Build history of the part. All positions in model axes, mm. A direction names the side the tool comes from. Give positions to 0.01 mm unless a question says otherwise; leave off trailing zeros. Order: outer loops, then holes, each group sorted by start corner. A loop starts at its lowest first (then second) coordinate and runs counter-clockwise, first axis right, second up. Notation, with made-up numbers: (16, 84) -> (71, 84) arc R33 cw to (71, 112) -> close; hole circle Ø9 at (-25, 27). An arc over 180 degrees is marked (long way). Use a Markdown table: item, result. Add a question column.
Autodesk Inventor part; units mm, degrees
ref_plane "YZ Plane" through (0, 0, 0) normal (1, 0, 0) x (0, 1, 0)
ref_plane "XZ Plane" through (0, 0, 0) normal (0, 1, 0) x (-1, 0, 0)
ref_plane "XY Plane" through (0, 0, 0) normal (0, 0, 1) x (1, 0, 0)
sketch "Sketch1" plane through (0, 0, 0) normal (0, 0, 1) x (1, 0, 0)
  circle A0 centre (-2.2725, 0) radius 4
  circle A1 centre (-2.2725, 0) radius 3.5
  point P0 (0, 0)
  dimension "d0" = 0.5
extrude "Extrusion1" add sketch "Sketch1" against normal blind 6 contours A1
sketch "Sketch2" plane through (-2.2725, 0, 0) normal (0, 0, 1) x (1, 0, 0)
  circle A0 centre (0, 0) radius 3.5
  arc A1 (0, 5) -> (0, -5) centre (0, 0) ccw
  line L0 (0, 5) -> (7.1657, 5)
  line L1 (0, -5) -> (7.1657, -5)
  line L2 (8.6657, 10) -> (7.1657, 10)
  line L3 (7.1657, -10) -> (8.6657, -10)
  line L4 (8.6657, -10) -> (8.6657, 10)
  line L5 (7.1657, 10) -> (7.1657, 5)
  line L6 (7.1657, -5) -> (7.1657, -10)
  point P0 (2.2725, 0)
  dimension "d3" = 10
  dimension "d5" = 20
  dimension "d6" = 5
  dimension "d7" = 5
  dimension "d8" = 1.5
  dimension "d11" = 1.5
extrude "Extrusion2" add sketch "Sketch2" along normal blind 5 contours A0 | L0 L5 L2 L4 L3 L6 L1 A1
sketch "Sketch3" plane through (-2.2725, 0, 0) normal (0, 0, -1) x (-1, 0, 0)
  arc A0 (0, -5) -> (0, 5) centre (0, 0) ccw
  line L0 (-7.1657, 5) -> (0, 5)
  line L1 (-7.1657, 10) -> (-7.1657, 5)
  line L2 (-8.6657, 10) -> (-7.1657, 10)
  line L3 (-8.6657, -10) -> (-8.6657, 10)
  line L4 (-7.1657, -10) -> (-8.6657, -10)
  line L5 (-7.1657, -5) -> (-7.1657, -10)
  line L6 (0, -5) -> (-7.1657, -5)
  circle A1 centre (0, 0) radius 3.5
  line L7 (-7.1657, -5) -> (-7.1657, -10)
  line L8 (-7.1657, -5) -> (-7.1657, 5)
  point P0 (-2.2725, 0)
extrude "Extrusion3" add sketch "Sketch3" along normal blind 15 contours L5 L4 L3 L2 L1 L8
fillet "Fillet1" radius 2 2 edges at (4.8932, 5, 2.5) (4.8932, -5, 2.5)
sketch "Sketch4" plane through (-2.2725, 0, -6) normal (0, 0, -1) x (-1, 0, 0)
  circle A0 centre (0, 0) radius 3.5
  point P0 (-2.2725, 0)
hole "Hole1" at (-2.2725, 0, -6) direction (0, 0, 1) diameter 3 end through all
equation "\"d7\" = d6"
equation "\"d11\" = d8"
properties part number "center_holder_boat"
(1) Wall check: probe 1 along X at (y, z) = (0, 0.75); probe 2 along X at (y, z) = (-8.5, -0.75); probe 3 along Y at (x, z) = (-3.25, -0.5). Give the ranges that are in metal, low to high.
(2) Band-saw the part on C-C on y = 0. Give the cut face in (x, z).
(3) Mould opens along X. For faces 1 (the face through (0, 5, 2)), 2 (the face through (-5.05, -2.13, -2.96)), 3 (the face through (4.32, -5.6, 2.54)) say: released by +X, released by -X, zero draft, split by the parting line, or undercut.
(4) Pin check, flat tips, straight feed: pin 1 Ø6 at (x, y) = (-2, 2.5) entering from -Z; pin 2 Ø3 at (x, z) = (-0.5, -4.5) entering from +Y; pin 3 Ø8 at (x, y) = (-4, -8) entering from +Z; pin 4 Ø1.5 at (x, z) = (0.5, 3) entering from +Y. Stop position of each tip, or through.
(5) Tool access for faces 4 (the face through (-2, -2, -6)), 5 (the face through (0, -5, 2)), 6 (the face through (1.4, 0.1, 0)): list every direction of +Z, -Z, +X, -X, +Y, -Y with a clear straight run to the whole face (end or side of a thin tool).
(6) Band-saw the part on A-A on z = -5.25. Give the cut face in (x, y).
(7) Band-saw the part on D-D on x = -3. Give the cut face in (y, z).
(8) Band-saw the part on B-B on z = 2.5. Give the cut face in (x, y), plus the area to 3 significant figures.
Response:
| question | item | result |
|---|---|---|
| 1 | probe 1 | x = -7.27 to -3.77, -0.77 to 6.39 |
| 1 | probe 2 | x = 4.89 to 6.39 |
| 1 | probe 3 | y = -3.36 to -1.14, 1.14 to 3.36 |
| 2 | outline | (-7.27, 0) -> (-5.77, 0) -> (-5.77, -6) -> (-3.77, -6) -> (-3.77, 5) -> (-7.27, 5) -> close; (-0.77, -6) -> (1.23, -6) -> (1.23, 0) -> (4.89, 0) -> (4.89, -15) -> (6.39, -15) -> (6.39, 5) -> (-0.77, 5) -> close |
| 3 | face 1 | zero draft |
| 3 | face 2 | undercut |
| 3 | face 3 | released by -X |
| 4 | pin 1 | stops at z = -6 |
| 4 | pin 2 | stops at y = 3.49 |
| 4 | pin 3 | stops at z = 5 |
| 4 | pin 4 | stops at y = 5 |
| 5 | face 4 | -Z, -X, +Y, -Y |
| 5 | face 5 | +Z, -Z, -X, -Y |
| 5 | face 6 | -Z |
| 6 | outline | circle Ø7 at (-2.27, 0); (4.89, -10) -> (6.39, -10) -> (6.39, 10) -> (4.89, 10) -> close; hole circle Ø3 at (-2.27, 0) |
| 7 | outline | (-4.95, 0) -> (-3.42, 0) -> (-3.42, -6) -> (-1.31, -6) -> (-1.31, 5) -> (-4.95, 5) -> close; (1.31, -6) -> (3.42, -6) -> (3.42, 0) -> (4.95, 0) -> (4.95, 5) -> (1.31, 5) -> close |
| 8 | outline | (-2.27, -5) -> (2.89, -5) arc R2 cw to (4.89, -7) -> (4.89, -10) -> (6.39, -10) -> (6.39, 10) -> (4.89, 10) -> (4.89, 7) arc R2 cw to (2.89, 5) -> (-2.27, 5) arc R5 ccw to start; hole circle Ø3 at (-2.27, 0) |
| 8 | area | 136 mm² |
